Here's how the part is built. I have some questions about the finished solid (model axes, mm). A direction names the side the tool comes from. Coordinates: 2 decimals unless noted, no trailing zeros. Loops run counter-clockwise (first coordinate to the right, second up) from the corner with the lowest first, then second, coordinate; pieces in that order, holes last. Notation, with made-up numbers: (-38, 52) -> (12, 52) arc R17 cw to (12, 57) -> close; hole circle Ø1 at (13.25, -10). An arc over 180 degrees is marked (long way). Answer as a JSON object with one key per item and string values. Group by question number.
1) I want a section at B-B (z = 9.5). Write out the boundary of the cut face in (x, y) (3 decimals).
2) Which directions (+Z, -Z, +X, -X, +Y, -Y) give clear straight access to the entire face, cutting with the end or side of a thin tool? Please do faces 4 (the flat face through (0, -8.76, -10)), 5 (the flat face through (9.22, -1, 22)), 6 (the flat face through (0, 0, 23)).
3) I want a section at C-C (x = -4.78). Write out the boundary of the cut face in (y, z) (3 decimals), then the cut area to 3 significant figures.
4) I want a section at D-D (z = -9.88). Write out the boundary of the cut face in (x, y) (3 decimals).
5) I want a section at A-A (y = 21.5). Write out the boundary of the cut face in (x, z) (3 decimals).
6) I need wall thicknesses on probe 1 along Y at (x, z) = (-5, 2); probe 2 along X at (y, z) = (-9, 5) (3 decimals); probe 3 along Z at (x, y) = (0, -14) (3 decimals). Which ranges of each line are inside material? Lowest first, please. Write a range as [from, to].
7) I'm going to push flat-ended pins straight in: pin 1 (4.5 mm diameter, centred on x = 4.78, z = 24.685, fed in from -Y); pin 2 (3.5 mm diameter, centred on x = -4.78, z = -24.685, fed in from +Y); pin 3 (2.5 mm diameter, centred on y = -1, z = -22, fed in from +X). Where does each tip first touch, or does it pass through?
8) If we mould it in two halves opening along Z, with no side actions, what happens to faces 1 (the cylindrical face through (-0.285, -12.816, -11.164)), 2 (the cylindrical face through (-8.6, -1.3, -26.1)), 3 (the cylindrical face through (8.6, -1.2, 26.1))? For each: +Z half, -Z half, draft (parallel to the pull), parting line (faces both ways), or undercut.
```python
from build123d import *

# Parameters (mm, degrees)
F0_W      = 19.81
F0_H      = 39.97
F1_DEPTH  = 8.94
F3_W      = 18.44
F3_H      = 2.47
F4_DEPTH  = 6.67
F2_W      = 18.44
F2_H      = 2.47
F5_DEPTH  = 6.67
F6_DEPTH  = 20.14
F8_DEPTH  = 1.98
F9_R      = 6.745
F10_DEPTH = 1
F11_R     = 5.48
F12_DEPTH = 1.2
F13_R     = 2.95
F14_DEPTH = 3.64
F15_R     = 1.315
F16_DEPTH = 8
F17_DEPTH = 6.23
F18_W     = 7.15
F18_H     = 3.8
F19_DEPTH = 8
F22_DEPTH = 5
F23_R     = 0.15
F24_R     = 2


with BuildPart() as f1:
    # F0 (on Front) → F1 (new body)
    with BuildSketch(Plane.XZ):
        Rectangle(F0_W, F0_H)
    extrude(amount=F1_DEPTH)

    # F3 (on face) → F4 (join)
    with BuildSketch(Plane(origin=(0, 0, -19.985), x_dir=(1, 0, 0), z_dir=(0, 0, -1))):
        with Locations((0, 1.235)):
            Rectangle(F3_W, F3_H)
    extrude(amount=F4_DEPTH)

    # F2 (on face) → F5 (join)
    with BuildSketch(Plane.XY.offset(19.985)):
        with Locations((0, -1.235)):
            Rectangle(F2_W, F2_H)
    extrude(amount=F5_DEPTH)

    # F0 (on Front) → F6 (join)
    with BuildSketch(Plane.XZ):
        Rectangle(F0_W, F0_H)
    extrude(amount=-F6_DEPTH)

    # F7 (on face) → F8 (join)
    with BuildSketch(Plane.XZ.offset(8.94)):
        with BuildLine():
            Line((0, -1.395), (-9.295, -1.395))
            Line((-9.295, -1.395), (-6.5725575311, -4.1174424689))
            ThreePointArc((-6.5725575311, -4.1174424689), (-3.5570425038, -2.1025397453), (0, -1.395))
        make_face()
        with BuildLine():
            Line((6.5725575311, -4.1174424689), (9.295, -1.395))
            Line((9.295, -1.395), (0, -1.395))
            ThreePointArc((0, -1.395), (3.5570425038, -2.1025397453), (6.5725575311, -4.1174424689))
        make_face()
        with BuildLine():
            Line((9.295, -10.69), (9.295, -1.395))
            Line((9.295, -1.395), (6.5725575311, -4.1174424689))
            ThreePointArc((6.5725575311, -4.1174424689), (8.5874602547, -7.1329574962), (9.295, -10.69))
        make_face()
        with BuildLine():
            ThreePointArc((-6.5725575311, -4.1174424689), (-8.5874602547, -7.1329574962), (-9.295, -10.69))
            Line((-9.295, -10.69), (0, -10.69))
            Line((0, -10.69), (-6.5725575311, -4.1174424689))
        make_face()
        with BuildLine():
            Line((0, -10.69), (-9.295, -10.69))
            ThreePointArc((-9.295, -10.69), (-8.5874602547, -14.2470425038), (-6.5725575311, -17.2625575311))
            Line((-6.5725575311, -17.2625575311), (0, -10.69))
        make_face()
        with BuildLine():
            Line((0, -19.985), (0, -10.69))
            Line((0, -10.69), (-6.5725575311, -17.2625575311))
            ThreePointArc((-6.5725575311, -17.2625575311), (-3.5570425038, -19.2774602547), (0, -19.985))
        make_face()
        with BuildLine():
            Line((6.5725575311, -17.2625575311), (0, -10.69))
            Line((0, -10.69), (0, -19.985))
            ThreePointArc((0, -19.985), (3.5570425038, -19.2774602547), (6.5725575311, -17.2625575311))
        make_face()
        with BuildLine():
            ThreePointArc((6.5725575311, -17.2625575311), (8.5874602547, -14.2470425038), (9.295, -10.69))
            Line((9.295, -10.69), (0, -10.69))
            Line((0, -10.69), (6.5725575311, -17.2625575311))
        make_face()
        with BuildLine():
            Line((0, -10.69), (9.295, -10.69))
            ThreePointArc((9.295, -10.69), (8.5874602547, -7.1329574962), (6.5725575311, -4.1174424689))
            Line((6.5725575311, -4.1174424689), (0, -10.69))
        make_face()
        with BuildLine():
            ThreePointArc((6.5725575311, -4.1174424689), (3.5570425038, -2.1025397453), (0, -1.395))
            ThreePointArc((0, -1.395), (-3.5570425038, -2.1025397453), (-6.5725575311, -4.1174424689))
            Line((-6.5725575311, -4.1174424689), (0, -10.69))
            Line((0, -10.69), (6.5725575311, -4.1174424689))
        make_face()
        Polygon((9.295, 14.875), (-9.295, 14.875), (-9.295, -1.395), (0, -1.395), (9.295, -1.395), align=None)
        with BuildLine():
            Line((-6.5725575311, -4.1174424689), (-9.295, -1.395))
            Line((-9.295, -1.395), (-9.295, -10.69))
            ThreePointArc((-9.295, -10.69), (-8.5874602547, -7.1329574962), (-6.5725575311, -4.1174424689))
        make_face()
    extrude(amount=F8_DEPTH)

    # F9 (on face) → F10 (join)
    with BuildSketch(Plane.XZ.offset(10.92)):
        with Locations((0, -9.88)):
            Circle(F9_R)
    extrude(amount=F10_DEPTH)

    # F11 (on face) → F12 (join)
    with BuildSketch(Plane.XZ.offset(11.92)):
        with Locations((0, -9.88)):
            Circle(F11_R)
    extrude(amount=F12_DEPTH)

    # F13 (on face) → F14 (join)
    with BuildSketch(Plane.XZ.offset(13.12)):
        with Locations((0, -9.88)):
            Circle(F13_R)
    extrude(amount=F14_DEPTH)

    # F15 (on face) → F16 (cut)
    with BuildSketch(Plane.XZ.offset(16.76)):
        with Locations((0, -9.88)):
            Circle(F15_R)
    extrude(amount=-F16_DEPTH, mode=Mode.SUBTRACT)

    # F17 (add): a face of the model
    f17_faces = [f1.faces().sort_by_distance(p)[0] for p in [
        (0, 20.14, 0),
    ]]
    extrude(f17_faces, amount=F17_DEPTH)

    # F18 (on face) → F19 (join)
    with BuildSketch(Plane(origin=(0, 0, -19.985), x_dir=(1, 0, 0), z_dir=(0, 0, -1))):
        with Locations((-0.14, -20.55)):
            Rectangle(F18_W, F18_H)
    extrude(amount=F19_DEPTH)

    # F20 (on face) + F21 (on face) → F22 (cut)
    with BuildSketch(Plane.XZ.offset(2.47)):
        with BuildLine():
            Line((5.1251086785, 26.655), (4.4348913215, 26.655))
            ThreePointArc((4.4348913215, 26.655), (3.4935742068, 23.1536252325), (6.78, 24.685))
            ThreePointArc((6.78, 24.685), (6.3113747675, 25.9714257932), (5.1251086785, 26.655))
        make_face()
        with BuildLine():
            ThreePointArc((-5.1251086785, 26.655), (-6.0664257932, 23.1536252325), (-2.78, 24.685))
            ThreePointArc((-2.78, 24.685), (-3.2486252325, 25.9714257932), (-4.4348913215, 26.655))
            Line((-4.4348913215, 26.655), (-5.1251086785, 26.655))
        make_face()
    with BuildSketch(Plane.XZ.offset(2.47)):
        with BuildLine():
            ThreePointArc((6.78, -24.685), (3.4935742068, -23.1536252325), (4.4348913215, -26.655))
            Line((4.4348913215, -26.655), (5.1251086785, -26.655))
            ThreePointArc((5.1251086785, -26.655), (6.3113747675, -25.9714257932), (6.78, -24.685))
        make_face()
        with BuildLine():
            ThreePointArc((-4.4348913215, -26.655), (-3.2486252325, -25.9714257932), (-2.78, -24.685))
            ThreePointArc((-2.78, -24.685), (-6.0664257932, -23.1536252325), (-5.1251086785, -26.655))
            Line((-5.1251086785, -26.655), (-4.4348913215, -26.655))
        make_face()
    extrude(amount=-F22_DEPTH, mode=Mode.SUBTRACT)

    # F23
    f23_edges = [f1.edges().sort_by_distance(p)[0] for p in [
        (-5.125109, -1.235, -26.655),
        (-4.434891, -1.235, -26.655),
        (4.434891, -1.235, -26.655),
        (5.125109, -1.235, -26.655),
        (5.125109, -1.235, 26.655),
        (-4.434891, -1.235, 26.655),
        (-5.125109, -1.235, 26.655),
        (4.434891, -1.235, 26.655),
    ]]
    fillet(f23_edges, radius=F23_R)

    # F24
    f24_edges = [f1.edges().sort_by_distance(p)[0] for p in [
        (9.22, -1.235, 26.655),
        (-9.22, -1.235, 26.655),
        (-9.22, -1.235, -26.655),
        (9.22, -1.235, -26.655),
    ]]
    fillet(f24_edges, radius=F24_R)


solid = f1.part
```
Determined:
{
 "1": {"outline": "(-9.905, -8.94) -> (-9.295, -8.94) -> (-9.295, -10.92) -> (9.295, -10.92) -> (9.295, -8.94) -> (9.905, -8.94) -> (9.905, 26.37) -> (-9.905, 26.37) -> close"},
 "2": {"face 4": "-Y", "face 5": "+Z, +X, +Y, -Y", "face 6": "+Z, +X, -X, +Y"},
 "3": {"outline": "(-13.12, -12.56) -> (-11.92, -12.56) -> (-11.92, -14.639) -> (-10.92, -14.639) -> (-10.92, -18.662) -> (-8.94, -18.662) -> (-8.94, -19.985) -> (-2.47, -19.985) -> (-2.47, -22.685) -> (0, -22.685) -> (0, -19.985) -> (26.37, -19.985) -> (26.37, 19.985) -> (0, 19.985) -> (0, 22.685) -> (-2.47, 22.685) -> (-2.47, 19.985) -> (-8.94, 19.985) -> (-8.94, 14.875) -> (-10.92, 14.875) -> (-10.92, -5.121) -> (-11.92, -5.121) -> (-11.92, -7.2) -> (-13.12, -7.2) -> close", "area": "1,510 mm^2"},
 "4": {"outline": "(-9.905, -8.94) -> (-9.295, -8.94) -> (-9.295, -10.92) -> (-6.745, -10.92) -> (-6.745, -11.92) -> (-5.48, -11.92) -> (-5.48, -13.12) -> (-2.95, -13.12) -> (-2.95, -16.76) -> (-1.315, -16.76) -> (-1.315, -8.76) -> (1.315, -8.76) -> (1.315, -16.76) -> (2.95, -16.76) -> (2.95, -13.12) -> (5.48, -13.12) -> (5.48, -11.92) -> (6.745, -11.92) -> (6.745, -10.92) -> (9.295, -10.92) -> (9.295, -8.94) -> (9.905, -8.94) -> (9.905, 26.37) -> (-9.905, 26.37) -> close"},
 "5": {"outline": "(-9.905, -19.985) -> (-3.715, -19.985) -> (-3.715, -27.985) -> (3.435, -27.985) -> (3.435, -19.985) -> (9.905, -19.985) -> (9.905, 19.985) -> (-9.905, 19.985) -> close"},
 "6": {"probe 1": "[-10.92, 26.37]", "probe 2": "[-9.295, 9.295]", "probe 3": "[-12.83, -11.195], [-8.565, -6.93]"},
 "7": {"pin 1": "y = -2.47", "pin 2": "y = 22.45", "pin 3": "x = 9.22"},
 "8": {"face 1": "undercut", "face 2": "-Z half", "face 3": "+Z half"}
}
